from build123d import *

# Parameters (mm, degrees)
SKETCH1_W               = 99
SKETCH1_H               = 88
SKETCH1_R               = 5
BOSS_EXTRUDE1_DEPTH     = 10
BOSS_EXTRUDE2_OUTLINE_R = 9.5
BOSS_EXTRUDE2_DEPTH     = 50
BOSS_EXTRUDE3_DEPTH     = 5
CUT_EXTRUDE3_DEPTH      = 10
FILLET1_R               = 13
FILLET2_R               = 13


# Read off the part's stored shape, not the designer's step: Boss-Extrude2
with BuildPart() as part:
    # Sketch1 → Boss-Extrude1 (new body)
    with BuildSketch(Plane(origin=(0, 0, 0), x_dir=(1, 0, 0), z_dir=(0, 1, 0))):
        with Locations((-3.690036969, 6.805517627)):
            Rectangle(SKETCH1_W, SKETCH1_H)
        with Locations(Location((-9.190036969, -18.194482373, 0), (0, 0, 270))):
            Circle(SKETCH1_R, mode=Mode.SUBTRACT)
        with Locations(Location((-9.190036969, 31.805517627, 0), (0, 0, 90))):
            Circle(SKETCH1_R, mode=Mode.SUBTRACT)
    extrude(amount=BOSS_EXTRUDE1_DEPTH)

    # Boss-Extrude2 outline → Boss-Extrude2 (add)
    with BuildSketch(Plane(origin=(0, 0, 0), x_dir=(1, 0, 0), z_dir=(0, 1, 0))):
        with BuildLine():
            ThreePointArc((-59.190036969, -12.203665814), (-54.947396282, -13.961025127), (-53.190036969, -18.203665814))
            Line((-53.190036969, -18.203665814), (-53.190036969, -37.203665814))
            Line((-53.190036969, -37.203665814), (-40.190036969, -37.203665814))
            Line((-40.190036969, -37.203665814), (-40.190036969, -15.203665814))
            ThreePointArc((-40.190036969, -15.203665814), (-39.311357313, -13.08234547), (-37.190036969, -12.203665814))
            Line((-37.190036969, -12.203665814), (-37.190036969, 1.796334186))
            Line((-37.190036969, 1.796334186), (-33.190036969, 1.796334186))
            Line((-33.190036969, 1.796334186), (-33.190036969, 11.796334186))
            Line((-33.190036969, 11.796334186), (-37.190036969, 11.796334186))
            Line((-37.190036969, 11.796334186), (-37.190036969, 25.796334186))
            ThreePointArc((-37.190036969, 25.796334186), (-39.311357313, 26.675013842), (-40.190036969, 28.796334186))
            Line((-40.190036969, 28.796334186), (-40.190036969, 50.796334186))
            Line((-40.190036969, 50.796334186), (-53.190036969, 50.796334186))
            Line((-53.190036969, 50.796334186), (-53.190036969, 31.796334186))
            ThreePointArc((-53.190036969, 31.796334186), (-54.947396282, 27.553693499), (-59.190036969, 25.796334186))
            ThreePointArc((-59.190036969, 25.796334186), (-78.190036969, 6.796334186), (-59.190036969, -12.203665814))
        make_face()
        with Locations((-59.190036969, 6.796334186)):
            Circle(BOSS_EXTRUDE2_OUTLINE_R, mode=Mode.SUBTRACT)
    extrude(amount=BOSS_EXTRUDE2_DEPTH)

    # 3DSketch2 → Boss-Extrude3 (add, symmetric)
    with BuildSketch(Plane(origin=(-33.190036969, 10, -6.796334186), x_dir=(1, 0, 0), z_dir=(0, 0, 1))):
        Polygon((0, 0), (60, 0), (0, 40), align=None)
    extrude(amount=BOSS_EXTRUDE3_DEPTH, both=True)

    # Sketch2 → Cut-Extrude3 (cut)
    with BuildSketch(Plane(origin=(0, 10, 0), x_dir=(1, 0, 0), z_dir=(0, 1, 0))):
        with BuildLine():
            ThreePointArc((38.793742347, 21.540492879), (43.966474405, 14.960601333), (45.809963031, 6.796430868))
            Line((45.809963031, 6.796430868), (45.809963031, 50.805517627))
            Line((45.809963031, 50.805517627), (2.809963031, 50.805517627))
            Line((2.809963031, 50.805517627), (38.793742347, 21.540492879))
        make_face()
        with BuildLine():
            Line((38.793742347, -7.947631063), (2.809963031, -37.194482373))
            Line((2.809963031, -37.194482373), (45.809963031, -37.194482373))
            Line((45.809963031, -37.194482373), (45.809963031, 6.796430868))
            ThreePointArc((45.809963031, 6.796430868), (43.966474387, -1.367739553), (38.793742347, -7.947631063))
        make_face()
    extrude(amount=-CUT_EXTRUDE3_DEPTH, mode=Mode.SUBTRACT)

    # Fillet1
    fillet1_edges = [part.edges().sort_by_distance(p)[0] for p in [
        (2.809963031, 5, 37.194482373),
    ]]
    fillet(fillet1_edges, radius=FILLET1_R)

    # Fillet2
    fillet2_edges = [part.edges().sort_by_distance(p)[0] for p in [
        (2.809963031, 5, -50.805517627),
    ]]
    fillet(fillet2_edges, radius=FILLET2_R)


solid = part.part
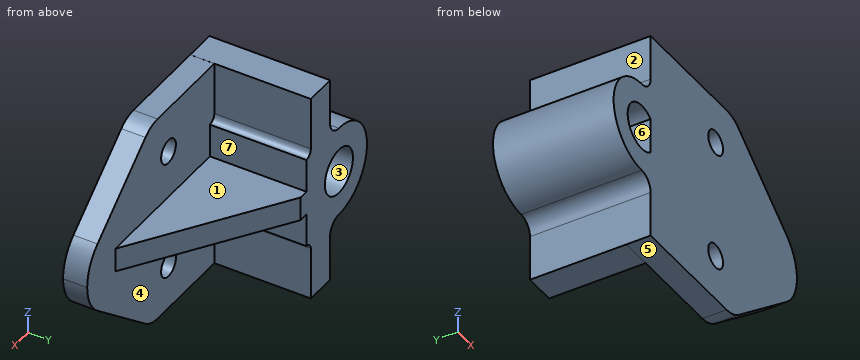
Build history of the part. All positions in model axes, mm. Face numbers are marked on the shaded views. A direction names the side the tool comes from. Coordinates: 2 decimals unless noted, no trailing zeros. Order: outer loops, then holes, each group sorted by start corner. A loop starts at its lowest first (then second) coordinate and runs counter-clockwise, first axis right, second up. Notation, with made-up numbers: (-1.5, 22.5) -> (51.5, 22.5) arc R19 ccw to (51.5, 57.5) -> close; hole circle Ø2 at (44.5, -33). An arc over 180 degrees is marked (long way). One line per item, written item: value.
(1) Mould opens along Z. For the marked faces 5, 6 and 7 say: pulls with the +Z half, pulls with the -Z half, needs draft (parallel to the pull), parting line crosses it, or undercut.
Checked values:
face 5: pulls with the -Z half
face 6: undercut
face 7: needs draft
(2) Slice it at A-A, the plane z = -9.5. List the corners of the cut face in (x, y), plus the area to 3 significant figures.
Checked values:
outline: (-78, 0) -> (-68.3, 0) -> (-68.3, 50) -> (-78, 50) -> close; (-53.19, 0) -> (45.62, 0) -> (45.62, 10) -> (26.81, 10) -> (-33.19, 50) -> (-50.08, 50) -> (-50.08, 10) -> (-53.19, 10) -> close
area: 3,350 mm2
(3) Slice it at D-D, the plane x = -35. List the corners of the cut face in (y, z).
Checked values:
outline: (0, -50.81) -> (10, -50.81) -> (10, -11.8) -> (50, -11.8) -> (50, -1.8) -> (10, -1.8) -> (10, 37.19) -> (0, 37.19) -> close
(4) Drop flat-ended pins along their axis: pin 1 Ø12 at (x, y) = (-4.5, 34) entering from +Z; pin 2 Ø4 at (x, z) = (-2.5, 19) entering from +Y; pin 3 Ø8 at (x, y) = (-26, 36) entering from -Z. Give the stop position or say it passes through.
Checked values:
pin 1: z = -1.8
pin 2: y = 10
pin 3: z = -11.8
(5) Tool access for the marked faces 1, 2, 3 and 4: list every direction of +Z, -Z, +X, -X, +Y, -Y with a clear straight run to the whole face (end or side of a thin tool).
Checked values:
face 1: +Z, +X, +Y
face 2: +Z, -X, +Y, -Y
face 3: +Y
face 4: +X, +Y
(6) Slice it at C-C, the plane y = 17. List the corners of the cut face in (x, z), plus the area to 3 significant figures.
Checked values:
outline: (-59.19, -25.8) arc R6 cw to (-53.19, -31.8) -> (-53.19, -50.8) -> (-40.19, -50.8) -> (-40.19, -28.8) arc R3 cw to (-37.19, -25.8) -> (-37.19, -11.8) -> (16.31, -11.8) -> (16.31, -1.8) -> (-37.19, -1.8) -> (-37.19, 12.2) arc R3 cw to (-40.19, 15.2) -> (-40.19, 37.2) -> (-53.19, 37.2) -> (-53.19, 18.2) arc R6 cw to (-59.19, 12.2) arc R19 ccw to start; hole circle Ø19 at (-59.19, -6.8)
area: 2,320 mm2
(7) Slice it at B-B, the plane x = -67. List the corners of the cut face in (y, z), plus the area to 3 significant figures.
Checked values:
outline: (0, -24.12) -> (50, -24.12) -> (50, -12.21) -> (0, -12.21) -> close; (0, -1.39) -> (50, -1.39) -> (50, 10.52) -> (0, 10.52) -> close
area: 1,190 mm2
(8) Probe line 1 (Z direction, x = -45, y = 29); line 2 (X direction, y = 36.5, z = -32.5); line 3 (Z direction, x = -19.5, y = 28.5). List the from-to ranges inside material, lowest first. Write a range as [from, to].
Checked values:
line 1: [-50.8, 37.2]
line 2: [-53.19, -40.19]
line 3: [-11.8, -1.8]
